```python
from build123d import *

# Parameters (mm, degrees)
F0_W     = 30.416689
F0_H     = 30.416687
F1_DEPTH = 12.5
F2_R     = 5.35
F3_DEPTH = 50


with BuildPart() as f1:
    # F0 (on Top) → F1 (new body, symmetric)
    with BuildSketch(Plane.XY):
        with Locations((-0.373975, -0.623292)):
            Rectangle(F0_W, F0_H)
    extrude(amount=F1_DEPTH, both=True)

    # F2 (on Front) → F3 (cut, symmetric)
    with BuildSketch(Plane.XZ):
        Circle(F2_R)
    extrude(amount=F3_DEPTH, both=True, mode=Mode.SUBTRACT)


solid = f1.part
```
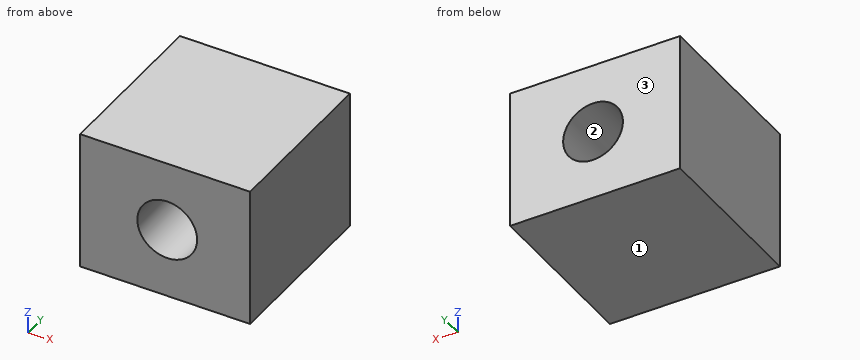
The model under review builds one solid part; all positions refer to its coordinate system, in mm. Face numbers are marked on the shaded views. Round coordinates to 2 decimals unless told otherwise and drop trailing zeros. Loops run counter-clockwise (first coordinate to the right, second up) from the corner with the lowest first, then second, coordinate; pieces in that order, holes last. Notation, with made-up numbers: (10.25, 5) -> (68.25, 5) arc R21 cw to (68.25, 31) -> close; hole circle Ø10 at (44.25, -29.5). An arc over 180 degrees is marked (long way). Answer as a JSON object with one key per item and string values. Group by question number.
1) We need section A-A on y = 1.5. Write out the cut boundary in (x, z), then the cut area to 3 significant figures.
2) For pin 1 Ø1.5 at (x, z) = (1, 5) entering from -Y; pin 2 Ø9.5 at (x, z) = (0, 0) entering from -Y, all flat-tipped, find the tip position at first contact; note any pin that passes through.
3) Mouldability with a two-part tool opening along Z and no side actions: class the marked faces 1, 2 and 3 as released by +Z, released by -Z, zero draft, split by the parting line, or undercut.
4) We need section C-C on x = 0. Write out the cut boundary in (y, z), then the cut area to 3 significant figures.
5) We need section B-B on z = 0. Write out the cut boundary in (x, y).
6) For line 1 (Z direction, x = 0, y = 3); line 2 (X direction, y = -1, z = 2.5); line 3 (X direction, y = 7.5, z = -3), list the stretches that pass through material, from the lowest coordinate up. Write a range as [from, to].
Result set:
{
 "1": {"outline": "(-15.58, -12.5) -> (14.83, -12.5) -> (14.83, 12.5) -> (-15.58, 12.5) -> close; hole circle Ø10.7 at (0, 0)", "area": "670 mm²"},
 "2": {"pin 1": "y = -15.83", "pin 2": "through"},
 "3": {"face 1": "released by -Z", "face 2": "undercut", "face 3": "zero draft"},
 "4": {"outline": "(-15.83, -12.5) -> (14.59, -12.5) -> (14.59, -5.35) -> (-15.83, -5.35) -> close; (-15.83, 5.35) -> (14.59, 5.35) -> (14.59, 12.5) -> (-15.83, 12.5) -> close", "area": "435 mm²"},
 "5": {"outline": "(-15.58, -15.83) -> (-5.35, -15.83) -> (-5.35, 14.59) -> (-15.58, 14.59) -> close; (5.35, -15.83) -> (14.83, -15.83) -> (14.83, 14.59) -> (5.35, 14.59) -> close"},
 "6": {"line 1": "[-12.5, -5.35], [5.35, 12.5]", "line 2": "[-15.58, -4.73], [4.73, 14.83]", "line 3": "[-15.58, -4.43], [4.43, 14.83]"}
}
